```python
from build123d import *

# Parameters (mm, degrees)
F0_R     = 1.778
F0_R_2   = 1.2446
F0_R_3   = 8.636
F1_DEPTH = 3.175
F2_R     = 8.89
F3_R     = 2.54


with BuildPart() as f1:
    # F0 (on Front) → F1 (new body)
    with BuildSketch(Plane.XZ):
        Polygon((24.638, -3.048), (24.638, 9.906), (-24.638, 9.906), (-24.638, -3.048), (-10.4775, -3.048), (-10.4775, -9.906), (10.4775, -9.906), (10.4775, -3.048), align=None)
        with Locations((-21.59, 0)):
            Circle(F0_R, mode=Mode.SUBTRACT)
        with Locations((-10.4775, 0)):
            Circle(F0_R_2, mode=Mode.SUBTRACT)
        Circle(F0_R_3, mode=Mode.SUBTRACT)
        with Locations((10.4775, 0)):
            Circle(F0_R_2, mode=Mode.SUBTRACT)
        with Locations((21.59, 0)):
            Circle(F0_R, mode=Mode.SUBTRACT)
    extrude(amount=F1_DEPTH)

    # F2
    f2_edges = [f1.edges().sort_by_distance(p)[0] for p in [
        (-24.638, -1.5875, 9.906),
        (24.638, -1.5875, 9.906),
    ]]
    fillet(f2_edges, radius=F2_R)

    # F3
    f3_edges = [f1.edges().sort_by_distance(p)[0] for p in [
        (-24.638, -1.5875, -3.048),
        (-10.4775, -1.5875, -3.048),
        (-10.4775, -1.5875, -9.906),
        (10.4775, -1.5875, -9.906),
        (24.638, -1.5875, -3.048),
        (10.4775, -1.5875, -3.048),
    ]]
    fillet(f3_edges, radius=F3_R)


solid = f1.part
```
Model file for the job. Use its own axes, mm. A direction names the side the tool comes from. Coordinates: 2 decimals unless noted, no trailing zeros. Write each loop counter-clockwise with the first axis right and the second up, starting at its lowest first coordinate (ties: lowest second). Pieces come first, ordered by that corner, then holes. Notation, with made-up numbers: (-34.75, 12.5) - (-25.75, 12.5) arc R35 ccw to (-25.75, 45.5) - close; hole circle Ø11 at (23, 18). An arc over 180 degrees is marked (long way). One line per question, with ' | ' between items. Start each with the question number.
Q1. Cut at A-A, the plane x = 0. List the corners of the cut face in (y, z) (3 decimals), then the cut area to 3 significant figures.
Q2. Pull direction Z, two halves, no side cores. Call faces 3 (the face through (-23.366, -1.565, 0.078)), 4 (the face through (22.103, -1.61, 7.233)), 5 (the face through (-10.478, -2, -6)), 6 (the face through (17, -2, -3.048)): pulls with the +Z half, pulls with the -Z half, needs draft (parallel to the pull), parting line crosses it, or undercut.
Q3. Cut at C-C, the plane y = -1.5. List the corners of the cut face in (x, z), then the cut area to 3 significant figures.
Q4. 3-axis set-ups, long thin cutter, end or side, ignore diameter. For faces 1 (the face through (10.478, -2, -6)), 2 (the face through (-24.638, -2, 0)): which of +Z, -Z, +X, -X, +Y, -Y reach the whole face in a straight line?
Q5. Cut at B-B, the plane z = 7.5. List the corners of the cut face in (x, y) (3 decimals).
Q6. Pin check, flat tips, straight feed: pin 1 (1.6 mm diameter, centred on x = 17, y = -1, fed in from -Z); pin 2 (4.5 mm diameter, centred on x = 21.59, z = 0, fed in from +Y); pin 3 (1 mm diameter, centred on y = -2.5, z = -5.5, fed in from -X); pin 4 (2 mm diameter, centred on x = -10.48, z = 0, fed in from -Y). Stop position of each tip, or through.
Q7. Cut at D-D, the plane x = -14. List the corners of the cut face in (y, z) (3 decimals), then the cut area to 3 significant figures.
Q8. Drill centre lines: line 1 (X direction, y = -0.5, z = 0.25); line 2 (Z direction, x = 21, y = -0.4); line 3 (Z direction, x = 21.59, y = -0.9). Where is each one in solid material? Low to high. Write a range as [from, to].
Answer below:
1) outline: (-3.175, -9.906) - (0, -9.906) - (0, -8.636) - (-3.175, -8.636) - close; (-3.175, 8.636) - (0, 8.636) - (0, 9.906) - (-3.175, 9.906) - close | area: 8.06 mm^2
2) face 3: undercut | face 4: pulls with the +Z half | face 5: needs draft | face 6: pulls with the -Z half
3) outline: (-24.64, -0.51) arc R2.54 ccw to (-22.1, -3.05) - (-13.02, -3.05) arc R2.54 cw to (-10.48, -5.59) - (-10.48, -7.37) arc R2.54 ccw to (-7.94, -9.91) - (7.94, -9.91) arc R2.54 ccw to (10.48, -7.37) - (10.48, -5.59) arc R2.54 cw to (13.02, -3.05) - (22.1, -3.05) arc R2.54 ccw to (24.64, -0.51) - (24.64, 1.02) arc R8.89 ccw to (15.75, 9.91) - (-15.75, 9.91) arc R8.89 ccw to (-24.64, 1.02) - close; hole circle Ø3.56 at (-21.59, 0); hole circle Ø2.49 at (-10.48, 0); hole circle Ø17.27 at (0, 0); hole circle Ø2.49 at (10.48, 0); hole circle Ø3.56 at (21.59, 0) | area: 481 mm^2
4) face 1: -Z, +X, +Y, -Y | face 2: +Z, -Z, -X, +Y, -Y
5) outline: (-21.83, -3.175) - (-4.281, -3.175) - (-4.281, 0) - (-21.83, 0) - close; (4.281, -3.175) - (21.83, -3.175) - (21.83, 0) - (4.281, 0) - close
6) pin 1: z = -3.05 | pin 2: y = 0 | pin 3: x = -10.55 | pin 4: through
7) outline: (-3.175, -3.048) - (0, -3.048) - (0, 9.906) - (-3.175, 9.906) - close | area: 41.1 mm^2
8) line 1: [-24.64, -23.35], [-19.83, -11.7], [-9.26, -8.63], [8.63, 9.26], [11.7, 19.83], [23.35, 24.64] | line 2: [-3.05, -1.68], [1.68, 8.19] | line 3: [-3.05, -1.78], [1.78, 7.72]
